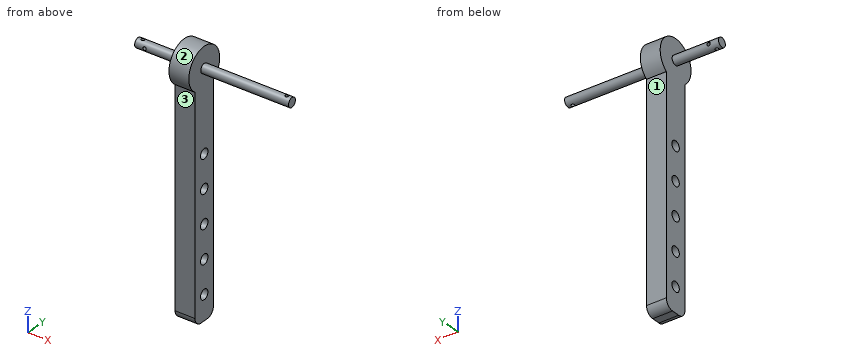
```python
from build123d import *

# Parameters (mm, degrees)
SKETCH_1_W           = 150
SKETCH_1_H           = 15
EXTRUDE_1_DEPTH      = 12
FILLET_1_R           = 5
SKETCH_6_R           = 12.5
EXTRUDE_2_DEPTH      = 12
EXTRUDE_5_DEPTH      = 28
EXTRUDE_5_DEPTH_BACK = 65
SKETCH_15_R          = 2.8
CUT_EXTRUDE_9_REACH  = 166.697
SKETCH_16_R          = 1
CUT_EXTRUDE_10_REACH = 166.697
SKETCH_17_R          = 3
SKETCH_18_R          = 1
CUT_EXTRUDE_11_DEPTH = 15


with BuildPart() as part:
    # 草图1 → 凸台-拉伸1 (new body)
    with BuildSketch(Plane(origin=(0, 0, 0), x_dir=(0, 0, -1), z_dir=(1, 0, 0))):
        with Locations((75, 7.5)):
            Rectangle(SKETCH_1_W, SKETCH_1_H)
    extrude(amount=EXTRUDE_1_DEPTH)

    # 圆角1
    fillet_1_edges = [part.edges().sort_by_distance(p)[0] for p in [
        (6, 15, 0),
        (6, 15, -150),
        (6, 0, -150),
        (6, 0, 0),
    ]]
    fillet(fillet_1_edges, radius=FILLET_1_R)

    # 草图6 → 凸台-拉伸2 (add)
    with BuildSketch(Plane(origin=(12, 0, 0), x_dir=(0, 0, -1), z_dir=(1, 0, 0))):
        with Locations((6.4, 7.5)):
            Circle(SKETCH_6_R)
    extrude(amount=-EXTRUDE_2_DEPTH)

    # 草图15 → 凸台-拉伸5 (add, two sides: drawn at the far end of the back side and taken through both)
    with BuildSketch(Plane.ZY.offset(-EXTRUDE_5_DEPTH_BACK)):
        with Locations((-6.4, 7.5)):
            Circle(SKETCH_15_R)
    extrude(amount=EXTRUDE_5_DEPTH + EXTRUDE_5_DEPTH_BACK)

    # 草图16 → 切除-拉伸9 (cut, up to next)
    with BuildSketch(Plane.XY, mode=Mode.PRIVATE) as cut_extrude_9_sk1:
        with Locations((-25, 7.5)):
            Circle(SKETCH_16_R)
    cut_extrude_9_tool1 = extrude(cut_extrude_9_sk1.sketch, amount=-CUT_EXTRUDE_9_REACH, mode=Mode.PRIVATE) & part.part
    # 草图16 → 切除-拉伸9 (cut, up to next)
    with BuildSketch(Plane.XY, mode=Mode.PRIVATE) as cut_extrude_9_sk2:
        with Locations((62, 7.5)):
            Circle(SKETCH_16_R)
    cut_extrude_9_tool2 = extrude(cut_extrude_9_sk2.sketch, amount=-CUT_EXTRUDE_9_REACH, mode=Mode.PRIVATE) & part.part
    add(cut_extrude_9_tool1.solids().sort_by_distance((-25, 7.5, 0))[0], mode=Mode.SUBTRACT)
    add(cut_extrude_9_tool2.solids().sort_by_distance((62, 7.5, 0))[0], mode=Mode.SUBTRACT)

    # 草图17 → 切除-拉伸10 (cut, up to next)
    with BuildSketch(Plane.ZY, mode=Mode.PRIVATE) as cut_extrude_10_sk1:
        with Locations((-135, 7.5)):
            Circle(SKETCH_17_R)
    cut_extrude_10_tool1 = extrude(cut_extrude_10_sk1.sketch, amount=-CUT_EXTRUDE_10_REACH, mode=Mode.PRIVATE) & part.part
    # 草图17 → 切除-拉伸10 (cut, up to next)
    with BuildSketch(Plane.ZY, mode=Mode.PRIVATE) as cut_extrude_10_sk2:
        with Locations((-115, 7.5)):
            Circle(SKETCH_17_R)
    cut_extrude_10_tool2 = extrude(cut_extrude_10_sk2.sketch, amount=-CUT_EXTRUDE_10_REACH, mode=Mode.PRIVATE) & part.part
    # 草图17 → 切除-拉伸10 (cut, up to next)
    with BuildSketch(Plane.ZY, mode=Mode.PRIVATE) as cut_extrude_10_sk3:
        with Locations((-95, 7.5)):
            Circle(SKETCH_17_R)
    cut_extrude_10_tool3 = extrude(cut_extrude_10_sk3.sketch, amount=-CUT_EXTRUDE_10_REACH, mode=Mode.PRIVATE) & part.part
    # 草图17 → 切除-拉伸10 (cut, up to next)
    with BuildSketch(Plane.ZY, mode=Mode.PRIVATE) as cut_extrude_10_sk4:
        with Locations((-75, 7.5)):
            Circle(SKETCH_17_R)
    cut_extrude_10_tool4 = extrude(cut_extrude_10_sk4.sketch, amount=-CUT_EXTRUDE_10_REACH, mode=Mode.PRIVATE) & part.part
    # 草图17 → 切除-拉伸10 (cut, up to next)
    with BuildSketch(Plane.ZY, mode=Mode.PRIVATE) as cut_extrude_10_sk5:
        with Locations((-55, 7.5)):
            Circle(SKETCH_17_R)
    cut_extrude_10_tool5 = extrude(cut_extrude_10_sk5.sketch, amount=-CUT_EXTRUDE_10_REACH, mode=Mode.PRIVATE) & part.part
    add(cut_extrude_10_tool1.solids().sort_by_distance((0, 7.5, -135))[0], mode=Mode.SUBTRACT)
    add(cut_extrude_10_tool2.solids().sort_by_distance((0, 7.5, -115))[0], mode=Mode.SUBTRACT)
    add(cut_extrude_10_tool3.solids().sort_by_distance((0, 7.5, -95))[0], mode=Mode.SUBTRACT)
    add(cut_extrude_10_tool4.solids().sort_by_distance((0, 7.5, -75))[0], mode=Mode.SUBTRACT)
    add(cut_extrude_10_tool5.solids().sort_by_distance((0, 7.5, -55))[0], mode=Mode.SUBTRACT)

    # 草图18 → 切除-拉伸11 (cut)
    with BuildSketch(Plane(origin=(0, 0, 0), x_dir=(1, 0, 0), z_dir=(0, 1, 0))):
        with Locations(Location((-22, 6.4, 0), (0, 0, 90))):
            Circle(SKETCH_18_R)
    extrude(amount=CUT_EXTRUDE_11_DEPTH, mode=Mode.SUBTRACT)


solid = part.part
```
The model under review builds one solid part; all positions refer to its coordinate system, in mm. Face numbers are marked on the shaded views. A direction names the side the tool comes from. Coordinates: 2 decimals unless noted, no trailing zeros. Order: outer loops, then holes, each group sorted by start corner. A loop starts at its lowest first (then second) coordinate and runs counter-clockwise, first axis right, second up. Notation, with made-up numbers: (81, 10.5) -> (102, 10.5) arc R38 ccw to (102, 48.5) -> close; hole circle Ø5 at (79.5, 42.5). An arc over 180 degrees is marked (long way). Answer in a Markdown table with one row per item. Add a question column.
Item 1: We need section D-D on y = 12.5. Write out the cut boundary in (x, z), plus the area to 3 significant figures.
Item 2: Clearance check with flat-ended pins moving along their axes: pin 1 (3.5 mm diameter, centred on x = 8.5, z = -111, fed in from -Y); pin 2 (8 mm diameter, centred on y = 7.5, z = -55, fed in from +X); pin 3 (1.8 mm diameter, centred on x = -22, z = -6.4, fed in from +Y); pin 4 (3.5 mm diameter, centred on x = 4, z = -77.5, fed in from +Y). State where each tip first meets the part, or that it passes through.
Item 3: To check wall thickness, follow probe 1 along Y at (x, z) = (7, -75); probe 2 along Z at (x, y) = (5, 9); probe 3 along Y at (x, z) = (5, -65.5). State the ranges of each line that lie inside material, in increasing order.
Item 4: We need section C-C on x = 15.5. Write out the cut boundary in (y, z), plus the area to 3 significant figures.
Item 5: Machinability: for the marked faces 1, 2 and 3, which of the approach directions +Z, -Z, +X, -X, +Y, -Y give a long, thin tool a straight path to every point of the face, cutting with its end or side? Answer none if there is none.
Item 6: We need section A-A on z = -95. Write out the cut boundary in (x, y), plus the area to 3 significant figures.
Item 7: We need section B-B on z = -74. Write out the cut boundary in (x, y).
Final values:
| question | item | result |
|---|---|---|
| 1 | outline | (0, -149.33) -> (12, -149.33) -> (12, 5.06) -> (0, 5.06) -> close |
| 1 | area | 1,850 mm2 |
| 2 | pin 1 | stops at y = 0 |
| 2 | pin 2 | stops at x = 12 |
| 2 | pin 3 | passes through |
| 2 | pin 4 | stops at y = 15 |
| 3 | probe 1 | y = 0 to 4.5, 10.5 to 15 |
| 3 | probe 2 | z = -150 to -137.6, -132.4 to -117.6, -112.4 to -97.6, -92.4 to -77.6, -72.4 to -57.6, -52.4 to 6.01 |
| 3 | probe 3 | y = 0 to 15 |
| 4 | outline | circle Ø5.6 at (7.5, -6.4) |
| 4 | area | 24.6 mm2 |
| 5 | face 1 | -Z, +X, -X, +Y |
| 5 | face 2 | +X, -X |
| 5 | face 3 | -Z, +X, -X, -Y |
| 6 | outline | (0, 0) -> (12, 0) -> (12, 4.5) -> (0, 4.5) -> close; (0, 10.5) -> (12, 10.5) -> (12, 15) -> (0, 15) -> close |
| 6 | area | 108 mm2 |
| 7 | outline | (0, 0) -> (12, 0) -> (12, 4.67) -> (0, 4.67) -> close; (0, 10.33) -> (12, 10.33) -> (12, 15) -> (0, 15) -> close |
